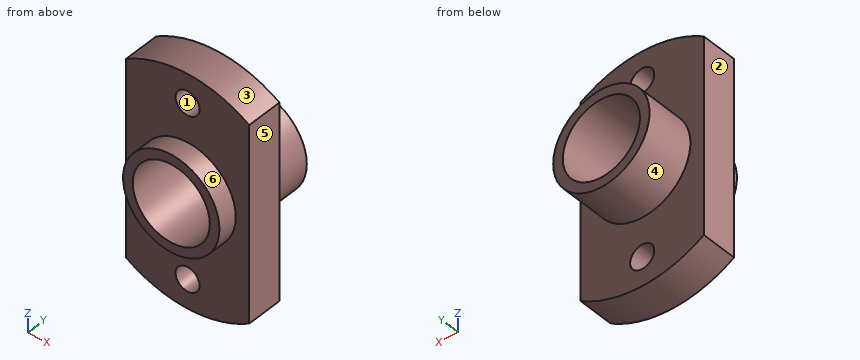
```python
from build123d import *

# Parameters (mm, degrees)
BOSS_EXTRUDE1_DEPTH      = 3.7
SKETCH2_R                = 5
BOSS_EXTRUDE2_DEPTH      = 5
BOSS_EXTRUDE2_DEPTH_BACK = 5.7
HOLE_WIZARD_M3_1_D       = 2.5
HOLE_WIZARD_M3_1_DEPTH   = 3.7
CUT_EXTRUDE_1_REACH      = 12.7
SKETCH_3_R               = 4


with BuildPart() as part:
    # Sketch1 → Boss-Extrude1 (new body)
    with BuildSketch(Plane(origin=(0, 0, 0), x_dir=(1, 0, 0), z_dir=(0, 1, 0))):
        with BuildLine():
            Line((-6.4, 10.150862032), (-6.4, -10.150862032))
            ThreePointArc((-6.4, -10.150862032), (0, -12), (6.4, -10.150862032))
            Line((6.4, -10.150862032), (6.4, 10.150862032))
            ThreePointArc((6.4, 10.150862032), (0, 12), (-6.4, 10.150862032))
        make_face()
    extrude(amount=BOSS_EXTRUDE1_DEPTH)

    # Sketch2 → Boss-Extrude2 (add, two sides)
    with BuildSketch(Plane(origin=(0, 3.7, 0), x_dir=(1, 0, 0), z_dir=(0, 1, 0))) as boss_extrude2_sk:
        Circle(SKETCH2_R)
    extrude(amount=BOSS_EXTRUDE2_DEPTH)
    extrude(boss_extrude2_sk.sketch, amount=-BOSS_EXTRUDE2_DEPTH_BACK)

    # M3 螺纹孔1
    with Locations(Plane(origin=(0, 0, 0), x_dir=(-1, 0, 0), z_dir=(0, -1, 0))):
        with Locations((0, -9), (0, 9)):
            Hole(HOLE_WIZARD_M3_1_D / 2, depth=HOLE_WIZARD_M3_1_DEPTH)

    # 草图3 → 切除-拉伸1 (cut, up to next)
    with BuildSketch(Plane.XZ.offset(2), mode=Mode.PRIVATE) as cut_extrude_1_sk1:
        Circle(SKETCH_3_R)
    cut_extrude_1_tool1 = extrude(cut_extrude_1_sk1.sketch, amount=-CUT_EXTRUDE_1_REACH, mode=Mode.PRIVATE) & part.part
    add(cut_extrude_1_tool1.solids().sort_by_distance((0, -2, 0))[0], mode=Mode.SUBTRACT)


solid = part.part
```
Read the model definition and answer for the solid it produces. Units are mm, in the model's axes. Face numbers are marked on the shaded views. A direction names the side the tool comes from. Give positions to 0.01 mm unless a question says otherwise; leave off trailing zeros. Write each loop counter-clockwise with the first axis right and the second up, starting at its lowest first coordinate (ties: lowest second). Pieces come first, ordered by that corner, then holes. Notation, with made-up numbers: M 88.5,-16 L 120.5,-16 A19 ccw 120.5,11 Z; hole C 83,64.5 d3. An arc over 180 degrees is marked long. Put each result on its own line as item: value. Start each with the question number.
1. Which of the six approach directions +Z, -Z, +X, -X, +Y, -Y give full straight-line access (tool end or side, diameter ignored) to the marked faces 4, 5 and 6?
2. Each of these flat-tipped pins is pushed along its axis until it touches: pin 1 Ø3 at (y, z) = (6, 1) entering from +X; pin 2 Ø1.5 at (x, y) = (-1.5, 4) entering from -Z. Where does it stop, or does it pass through?
3. The part is cut by section D-D, the plane x = 3. Give the vertices of the cut face in (y, z).
4. Consider line 1 along Z through (x, y) = (-1, 2.25); line 2 along X through (y, z) = (1.95, 9); line 3 along Y through (x, z) = (1.75, -7.25). Determine where each line is inside the solid, lowest interval first.
5. The part is cut by section C-C, the plane y = 1.75. Give the vertices of the cut face in (x, z), and give its area (3 significant figures).
6. For a pull along Z with two mould halves and no side action, classify the marked faces 1, 2 and 3 as released by +Z, released by -Z, zero draft, split by the parting line, or undercut.
7. The part is cut by section A-A, the plane x = 0. Give the vertices of the cut face in (y, z), and give its area (3 significant figures).
8. The part is cut by section B-B, the plane z = 0. Give the vertices of the cut face in (x, y), and give its area (3 significant figures).
Final values:
1. face 4: +Y
1. face 5: +Z, -Z, +X, +Y, -Y
1. face 6: -Y
2. pin 1: stops at x = 5
2. pin 2: stops at z = -11.97
3. outline: M -2,-4 L 0,-4 L 0,-11.62 L 3.7,-11.62 L 3.7,-4 L 8.7,-4 L 8.7,-2.65 L -2,-2.65 Z; M -2,2.65 L 8.7,2.65 L 8.7,4 L 3.7,4 L 3.7,11.62 L 0,11.62 L 0,4 L -2,4 Z
4. line 1: z = -11.96 to -9.75, -8.25 to -3.87, 3.87 to 8.25, 9.75 to 11.96
4. line 2: x = -6.4 to -1.25, 1.25 to 6.4
4. line 3: y = 0 to 3.7
5. outline: M -6.4,-10.15 A12 ccw 6.4,-10.15 L 6.4,10.15 A12 ccw -6.4,10.15 Z; hole C 0,0 d8; hole C 0,-9 d2.5; hole C 0,9 d2.5
5. area: 232 mm²
6. face 1: undercut
6. face 2: zero draft
6. face 3: released by +Z
7. outline: M -2,-5 L 0,-5 L 0,-7.75 L 3.7,-7.75 L 3.7,-5 L 8.7,-5 L 8.7,-4 L -2,-4 Z; M -2,4 L 8.7,4 L 8.7,5 L 3.7,5 L 3.7,7.75 L 0,7.75 L 0,5 L -2,5 Z; M 0,-12 L 3.7,-12 L 3.7,-10.25 L 0,-10.25 Z; M 0,10.25 L 3.7,10.25 L 3.7,12 L 0,12 Z
7. area: 54.7 mm²
8. outline: M -6.4,0 L -5,0 L -5,-2 L -4,-2 L -4,8.7 L -5,8.7 L -5,3.7 L -6.4,3.7 Z; M 4,-2 L 5,-2 L 5,0 L 6.4,0 L 6.4,3.7 L 5,3.7 L 5,8.7 L 4,8.7 Z
8. area: 31.8 mm²
